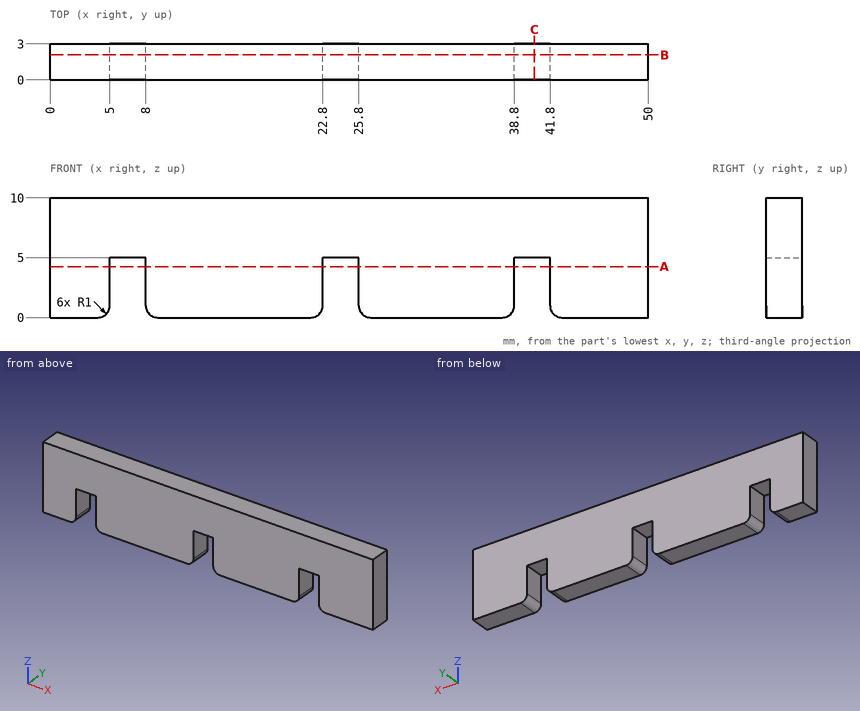
Input: dimensioned drawing with shaded views. Units: mm. Origin: part minimum x, y, z. Round coordinates to 2 decimals unless told otherwise and drop trailing zeros. Order: outer loops, then holes, each group sorted by start corner. A loop starts at its lowest first (then second) coordinate and runs counter-clockwise, first axis right, second up.
1. Cut plane B-B, the plane y = 2.1. Output: boundary loops of the cut face in (x, z), then the cut area to 3 significant figures.
The answers:
outline: (0, 0) - (4, 0) arc R1 ccw to (5, 1) - (5, 5) - (8, 5) - (8, 1) arc R1 ccw to (9, 0) - (21.8, 0) arc R1 ccw to (22.8, 1) - (22.8, 5) - (25.8, 5) - (25.8, 1) arc R1 ccw to (26.8, 0) - (37.8, 0) arc R1 ccw to (38.8, 1) - (38.8, 5) - (41.8, 5) - (41.8, 1) arc R1 ccw to (42.8, 0) - (50, 0) - (50, 10) - (0, 10) - close
area: 454 mm2
2. Cut plane A-A, the plane z = 4.25. Output: boundary loops of the cut face in (x, y).
The answers:
outline: (0, 0) - (5, 0) - (5, 3) - (0, 3) - close; (8, 0) - (22.8, 0) - (22.8, 3) - (8, 3) - close; (25.8, 0) - (38.8, 0) - (38.8, 3) - (25.8, 3) - close; (41.8, 0) - (50, 0) - (50, 3) - (41.8, 3) - close
3. Cut plane C-C, the plane x = 40.5. Output: boundary loops of the cut face in (y, z), then the cut area to 3 significant figures.
The answers:
outline: (0, 5) - (3, 5) - (3, 10) - (0, 10) - close
area: 15.0 mm2
4. Pin query (flat end, axial travel): P1, Ø1.5, axis at x = 24.5, y = 1.5, coming from the -Z side. Return the tip coordinate at first contact, or that it passes through.
The answers:
P1: stops at z = 5
5. Material intervals for line 1 (X direction, y = 2.1, z = 1); line 2 (X direction, y = 2.5, z = 0.5); line 3 (Z direction, x = 25, y = 1.75), sorted ascending.
The answers:
line 1: x = 0 to 5, 8 to 22.8, 25.8 to 38.8, 41.8 to 50
line 2: x = 0 to 4.87, 8.13 to 22.67, 25.93 to 38.67, 41.93 to 50
line 3: z = 5 to 10
